from build123d import *

# Parameters (mm, degrees)
PER_AGE1_D           = 3
PER_AGE1_CBORE_D     = 5
PER_AGE1_CBORE_DEPTH = 3


with BuildPart() as part:
    # Esquisse1 → Révolution1 (revolve)
    with BuildSketch(Plane(origin=(0, 0, 0), x_dir=(0, 0, -1), z_dir=(1, 0, 0))):
        Polygon((0, 2), (-15, 2), (-15, 1), (-13, 1), (-13, -1), (-15, -1), (-15, -2), (0, -2), align=None)
    revolve(axis=Axis((0, 2, 0), (0, -1, 0)))

    # Perçage1 (through all)
    with Locations(Plane(origin=(0, 2, 0), x_dir=(1, 0, 0), z_dir=(0, 1, 0))):
        with Locations((0, 0)):
            CounterBoreHole(PER_AGE1_D / 2, PER_AGE1_CBORE_D / 2, PER_AGE1_CBORE_DEPTH)


solid = part.part
Work out the finished part from the listing and answer in its coordinate system (mm). A direction names the side the tool comes from. Round coordinates to 2 decimals unless told otherwise and drop trailing zeros. Write each loop counter-clockwise with the first axis right and the second up, starting at its lowest first coordinate (ties: lowest second). Pieces come first, ordered by that corner, then holes. Notation, with made-up numbers: (-27, 16) - (5, 16) arc R37 ccw to (5, 54) - close; hole circle Ø7 at (55, -22.75). An arc over 180 degrees is marked (long way). Answer in a Markdown table with one row per item. Add a question column.
1. Given pin 1 (1.5 mm diameter, centred on y = 1, z = 6, fed in from -X); pin 2 (8 mm diameter, centred on x = 0, z = 0, fed in from -Y); pin 3 (1.5 mm diameter, centred on y = 0.5, z = -7, fed in from +X); pin 4 (2.5 mm diameter, centred on x = -0.5, z = -0.5, fed in from +Y), each flat-ended and moving along its own axis, determine where each tip first touches the part or whether it passes through.
2. A cutting plane is placed at D-D, the plane x = 9. Determine the outline of the cut face in (y, z).
3. Find the intervals of material crossed by line 1 along Z through (x, y) = (0, -1.5); line 2 along Z through (x, y) = (0, 0.1); line 3 along Y through (x, z) = (-4.25, 12.75), in increasing order. Write a range as from..to.
4. A cutting plane is placed at B-B, the plane x = 0. Determine the outline of the cut face in (y, z).
5. A cutting plane is placed at A-A, the plane z = 0. Determine the outline of the cut face in (x, y), and give its area (3 significant figures).
6. The mould has two halves that part along Y. Classify faces 4 (the flat face through (3, -2, 0)), 5 (the cylindrical face through (-0.54, 0.52, 2.44)), 6 (the cylindrical face through (7.91, -0.014, -10.316)): +Y half, -Y half, draft (parallel to the pull), parting line (faces both ways), or undercut.
7. For faces 1 (the flat face through (2, -1, 0)), 2 (the flat face through (-13.4, 1, -0.1)), 3 (the cylindrical face through (1.5, -1.51, -0.07)), determine the directions among +Z, -Z, +X, -X, +Y, -Y from which every point of the face is accessible in a straight line to the end or side of a thin tool.
8. A cutting plane is placed at C-C, the plane y = -1.45. Determine the outline of the cut face in (x, z).
Worked out:
| question | item | result |
|---|---|---|
| 1 | pin 1 | x = -14.05 |
| 1 | pin 2 | y = -2 |
| 1 | pin 3 | x = 13.55 |
| 1 | pin 4 | y = -1 |
| 2 | outline | (-2, -12) - (-1, -12) - (-1, -9.38) - (1, -9.38) - (1, -12) - (2, -12) - (2, 12) - (1, 12) - (1, 9.38) - (-1, 9.38) - (-1, 12) - (-2, 12) - close |
| 3 | line 1 | -15..-1.5, 1.5..15 |
| 3 | line 2 | -13..-2.5, 2.5..13 |
| 3 | line 3 | -2..-1, 1..2 |
| 4 | outline | (-2, -15) - (-1, -15) - (-1, -13) - (1, -13) - (1, -15) - (2, -15) - (2, -2.5) - (-1, -2.5) - (-1, -1.5) - (-2, -1.5) - close; (-2, 1.5) - (-1, 1.5) - (-1, 2.5) - (2, 2.5) - (2, 15) - (1, 15) - (1, 13) - (-1, 13) - (-1, 15) - (-2, 15) - close |
| 5 | outline | (-15, -2) - (-1.5, -2) - (-1.5, -1) - (-2.5, -1) - (-2.5, 2) - (-15, 2) - (-15, 1) - (-13, 1) - (-13, -1) - (-15, -1) - close; (1.5, -2) - (15, -2) - (15, -1) - (13, -1) - (13, 1) - (15, 1) - (15, 2) - (2.5, 2) - (2.5, -1) - (1.5, -1) - close |
| 5 | area | 94.0 mm^2 |
| 6 | face 4 | -Y half |
| 6 | face 5 | draft |
| 6 | face 6 | undercut |
| 7 | face 1 | +Y |
| 7 | face 2 | none |
| 7 | face 3 | +Y, -Y |
| 8 | outline | circle Ø30 at (0, 0); hole circle Ø3 at (0, 0) |
